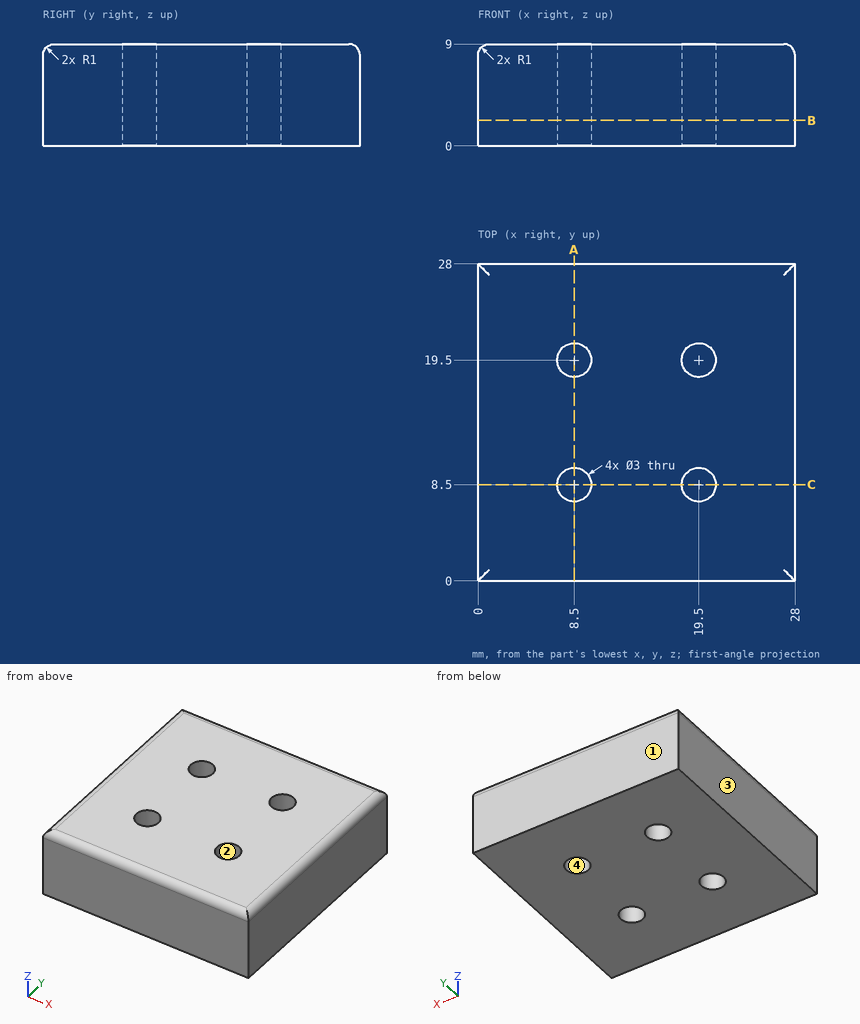
Verification items for this drawing (mm, ordinates from the low corner). Give positions to 0.01 mm unless a question says otherwise; leave off trailing zeros. Order: outer loops, then holes, each group sorted by start corner. A loop starts at its lowest first (then second) coordinate and runs counter-clockwise, first axis right, second up.
1) Draft check along Y on the marked faces 1, 2, 3 and 4. Enter one of: released by +Y, released by -Y, zero draft, split by the parting line, or undercut.
Results are:
face 1: released by +Y
face 2: undercut
face 3: zero draft
face 4: undercut
2) Gauge pin test, flat ends, axial feed: pin 1 (2.5 mm diameter, centred on x = 8.5, y = 8.5, fed in from +Z); pin 2 (5 mm diameter, centred on x = 8.5, y = 19.5, fed in from +Z). Record the tip position at first contact, or that the pin passes through.
Results are:
pin 1: passes through
pin 2: stops at z = 9
3) Material ranges on probe 1 along Y at (x, z) = (8.5, 2); probe 2 along X at (y, z) = (8, 5); probe 3 along Y at (x, z) = (7.25, 5), recorded low to high.
Results are:
probe 1: y = 0 to 7, 10 to 18, 21 to 28
probe 2: x = 0 to 7.09, 9.91 to 18.09, 20.91 to 28
probe 3: y = 0 to 7.67, 9.33 to 18.67, 20.33 to 28
4) Cross-section at B-B (z = 2.25). Record the boundary of the cut face in (x, y), then the cut area to 3 significant figures.
Results are:
outline: (0, 0) - (28, 0) - (28, 28) - (0, 28) - close; hole circle Ø3 at (8.5, 8.5); hole circle Ø3 at (8.5, 19.5); hole circle Ø3 at (19.5, 8.5); hole circle Ø3 at (19.5, 19.5)
area: 756 mm2
5) Cross-section at A-A (x = 8.5). Record the boundary of the cut face in (y, z).
Results are:
outline: (0, 0) - (7, 0) - (7, 9) - (1, 9) arc R1 ccw to (0, 8) - close; (10, 0) - (18, 0) - (18, 9) - (10, 9) - close; (21, 0) - (28, 0) - (28, 8) arc R1 ccw to (27, 9) - (21, 9) - close
